```python
from build123d import *

# Parameters (mm, degrees)
EXTRUDE_1_DEPTH          = 5
EXTRUDE_1_DEPTH_BACK     = 5
SKETCH_1_R               = 45
CUT_EXTRUDE_1_DEPTH      = 64.835726674
CUT_EXTRUDE_1_DEPTH_BACK = 64.835726674
SKETCH_2_R               = 3


with BuildPart() as part:
    # 草图1 → 凸台-拉伸1 (new, two sides: drawn at the far end of the back side and taken through both)
    with BuildSketch(Plane.XY.offset(-EXTRUDE_1_DEPTH_BACK)):
        Circle(SKETCH_1_R)
        with BuildLine():
            Line((29.8555418, 2.94051421), (34.831465434, 3.430599912))
            ThreePointArc((34.831465434, 3.430599912), (35, 0), (34.831465434, -3.430599912))
            Line((34.831465434, -3.430599912), (29.8555418, -2.94051421))
            ThreePointArc((29.8555418, -2.94051421), (29.423558412, -5.85270966), (28.708210072, -8.708540318))
            Line((28.708210072, -8.708540318), (33.492911751, -10.159963704))
            ThreePointArc((33.492911751, -10.159963704), (32.335783638, -13.393920133), (30.867244252, -16.498885789))
            Line((30.867244252, -16.498885789), (26.45763793, -14.141902105))
            ThreePointArc((26.45763793, -14.141902105), (24.944088369, -16.667106991), (23.190313601, -19.031798525))
            Line((23.190313601, -19.031798525), (27.055365868, -22.203764946))
            ThreePointArc((27.055365868, -22.203764946), (24.748737342, -24.748737342), (22.203764946, -27.055365868))
            Line((22.203764946, -27.055365868), (19.031798525, -23.190313601))
            ThreePointArc((19.031798525, -23.190313601), (16.667106991, -24.944088369), (14.141902105, -26.45763793))
            Line((14.141902105, -26.45763793), (16.498885789, -30.867244252))
            ThreePointArc((16.498885789, -30.867244252), (13.393920133, -32.335783638), (10.159963704, -33.492911751))
            Line((10.159963704, -33.492911751), (8.708540318, -28.708210072))
            ThreePointArc((8.708540318, -28.708210072), (5.85270966, -29.423558412), (2.94051421, -29.8555418))
            Line((2.94051421, -29.8555418), (3.430599912, -34.831465434))
            ThreePointArc((3.430599912, -34.831465434), (0, -35), (-3.430599912, -34.831465434))
            Line((-3.430599912, -34.831465434), (-2.94051421, -29.8555418))
            ThreePointArc((-2.94051421, -29.8555418), (-5.85270966, -29.423558412), (-8.708540318, -28.708210072))
            Line((-8.708540318, -28.708210072), (-10.159963704, -33.492911751))
            ThreePointArc((-10.159963704, -33.492911751), (-13.393920133, -32.335783638), (-16.498885789, -30.867244252))
            Line((-16.498885789, -30.867244252), (-14.141902105, -26.45763793))
            ThreePointArc((-14.141902105, -26.45763793), (-16.667106991, -24.944088369), (-19.031798525, -23.190313601))
            Line((-19.031798525, -23.190313601), (-22.203764946, -27.055365868))
            ThreePointArc((-22.203764946, -27.055365868), (-24.748737342, -24.748737342), (-27.055365868, -22.203764946))
            Line((-27.055365868, -22.203764946), (-23.190313601, -19.031798525))
            ThreePointArc((-23.190313601, -19.031798525), (-24.944088369, -16.667106991), (-26.45763793, -14.141902105))
            Line((-26.45763793, -14.141902105), (-30.867244252, -16.498885789))
            ThreePointArc((-30.867244252, -16.498885789), (-32.335783638, -13.393920133), (-33.492911751, -10.159963704))
            Line((-33.492911751, -10.159963704), (-28.708210072, -8.708540318))
            ThreePointArc((-28.708210072, -8.708540318), (-29.423558412, -5.85270966), (-29.8555418, -2.94051421))
            Line((-29.8555418, -2.94051421), (-34.831465434, -3.430599912))
            ThreePointArc((-34.831465434, -3.430599912), (-35, 0), (-34.831465434, 3.430599912))
            Line((-34.831465434, 3.430599912), (-29.8555418, 2.94051421))
            ThreePointArc((-29.8555418, 2.94051421), (-29.423558412, 5.85270966), (-28.708210072, 8.708540318))
            Line((-28.708210072, 8.708540318), (-33.492911751, 10.159963704))
            ThreePointArc((-33.492911751, 10.159963704), (-32.335783638, 13.393920133), (-30.867244252, 16.498885789))
            Line((-30.867244252, 16.498885789), (-26.45763793, 14.141902105))
            ThreePointArc((-26.45763793, 14.141902105), (-24.944088369, 16.667106991), (-23.190313601, 19.031798525))
            Line((-23.190313601, 19.031798525), (-27.055365868, 22.203764946))
            ThreePointArc((-27.055365868, 22.203764946), (-24.748737342, 24.748737342), (-22.203764946, 27.055365868))
            Line((-22.203764946, 27.055365868), (-19.031798525, 23.190313601))
            ThreePointArc((-19.031798525, 23.190313601), (-16.667106991, 24.944088369), (-14.141902105, 26.45763793))
            Line((-14.141902105, 26.45763793), (-16.498885789, 30.867244252))
            ThreePointArc((-16.498885789, 30.867244252), (-13.393920133, 32.335783638), (-10.159963704, 33.492911751))
            Line((-10.159963704, 33.492911751), (-8.708540318, 28.708210072))
            ThreePointArc((-8.708540318, 28.708210072), (-5.85270966, 29.423558412), (-2.94051421, 29.8555418))
            Line((-2.94051421, 29.8555418), (-3.430599912, 34.831465434))
            ThreePointArc((-3.430599912, 34.831465434), (0, 35), (3.430599912, 34.831465434))
            Line((3.430599912, 34.831465434), (2.94051421, 29.8555418))
            ThreePointArc((2.94051421, 29.8555418), (5.85270966, 29.423558412), (8.708540318, 28.708210072))
            Line((8.708540318, 28.708210072), (10.159963704, 33.492911751))
            ThreePointArc((10.159963704, 33.492911751), (13.393920133, 32.335783638), (16.498885789, 30.867244252))
            Line((16.498885789, 30.867244252), (14.141902105, 26.45763793))
            ThreePointArc((14.141902105, 26.45763793), (16.667106991, 24.944088369), (19.031798525, 23.190313601))
            Line((19.031798525, 23.190313601), (22.203764946, 27.055365868))
            ThreePointArc((22.203764946, 27.055365868), (24.748737342, 24.748737342), (27.055365868, 22.203764946))
            Line((27.055365868, 22.203764946), (23.190313601, 19.031798525))
            ThreePointArc((23.190313601, 19.031798525), (24.944088369, 16.667106991), (26.45763793, 14.141902105))
            Line((26.45763793, 14.141902105), (30.867244252, 16.498885789))
            ThreePointArc((30.867244252, 16.498885789), (32.335783638, 13.393920133), (33.492911751, 10.159963704))
            Line((33.492911751, 10.159963704), (28.708210072, 8.708540318))
            ThreePointArc((28.708210072, 8.708540318), (29.423558412, 5.85270966), (29.8555418, 2.94051421))
        make_face(mode=Mode.SUBTRACT)
    extrude(amount=EXTRUDE_1_DEPTH + EXTRUDE_1_DEPTH_BACK)

    # 草图2 → 切除-拉伸1 (cut, two sides: drawn at the far end of the back side and taken through both)
    with BuildSketch(Plane.XY.offset(-CUT_EXTRUDE_1_DEPTH_BACK)):
        with Locations((40, 0)):
            Circle(SKETCH_2_R)
        with Locations((0, -40)):
            Circle(SKETCH_2_R)
        with Locations((-40, 0)):
            Circle(SKETCH_2_R)
        with Locations((0, 40)):
            Circle(SKETCH_2_R)
    extrude(amount=CUT_EXTRUDE_1_DEPTH + CUT_EXTRUDE_1_DEPTH_BACK, mode=Mode.SUBTRACT)


solid = part.part
```
CAD build for the part. Positions are in the model's coordinates, mm. Give positions to 0.01 mm unless a question says otherwise; leave off trailing zeros. Loops run counter-clockwise (first coordinate to the right, second up) from the corner with the lowest first, then second, coordinate; pieces in that order, holes last. Notation, with made-up numbers: M -19,8 L 15,8 A24 cw 15,26 Z; hole C -23.5,-6.75 d1. An arc over 180 degrees is marked long. Use one line per item in the form item = value.
Item 1: Drill centre lines: probe 1 along Y at (x, z) = (0, -2.5); probe 2 along Y at (x, z) = (30, -0.5); probe 3 along X at (y, z) = (26, 0.75). Where is each one in solid material? Low to high. Write a range as from..to.
Determined:
probe_1 = -45..-43, -37..-35, 35..37, 43..45
probe_2 = -33.54..-16.04, -9.1..-2.95, 2.95..9.1, 16.04..33.54
probe_3 = -36.73..-23.43, -21.34..-14.97, 14.97..21.34, 23.43..36.73
Item 2: Flat gauge pins, fed straight in: pin 1 (3 mm diameter, centred on y = 31.5, z = 1, fed in from -X); pin 2 (5.5 mm diameter, centred on x = 40, y = 0, fed in from -Z); pin 3 (5 mm diameter, centred on x = 30, z = 2.5, fed in from -Y); pin 4 (3 mm diameter, centred on y = 25.5, z = -2.5, fed in from +X). Where does each tip first touch, or does it go through?
Determined:
pin_1 = -33.54
pin_2 = through
pin_3 = -35.62
pin_4 = 38.07
Item 3: Slice it at C-C (x = 40). List the corners of the cut face in (y, z).
Determined:
outline = M -20.62,-5 L -3,-5 L -3,5 L -20.62,5 Z; M 3,-5 L 20.62,-5 L 20.62,5 L 3,5 Z
Item 4: Two-plate mould, pull along X, no slides. Class faces 1 (the face through (-25.1, -20.6, -0.1)), 2 (the face through (6, -30, -5)), 3 (the face through (20.6, -25.1, -0.1)): pulls with the +X half, pulls with the -X half, needs draft (parallel to the pull), parting line crosses it, or undercut.
Determined:
face_1 = undercut
face_2 = needs draft
face_3 = undercut
Item 5: Slice it at A-A (x = 0). List the corners of the cut face in (y, z), plus the area to 3 significant figures.
Determined:
outline = M -45,-5 L -43,-5 L -43,5 L -45,5 Z; M -37,-5 L -35,-5 L -35,5 L -37,5 Z; M 35,-5 L 37,-5 L 37,5 L 35,5 Z; M 43,-5 L 45,-5 L 45,5 L 43,5 Z
area = 80.0 mm2
